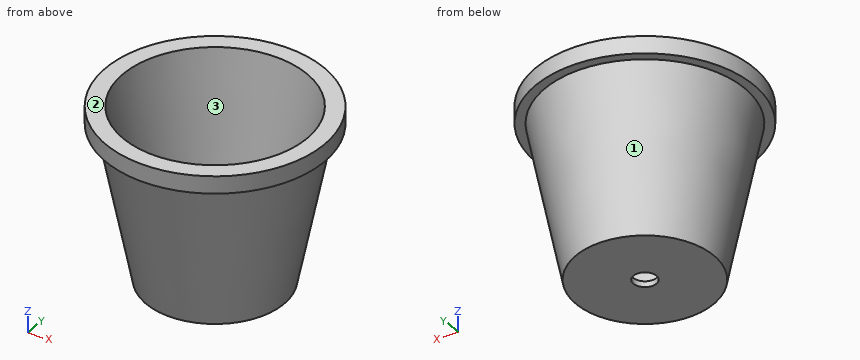
```python
from build123d import *

# Parameters (mm, degrees)
SKETCH_R      = 10
POCKET_DEPTH  = 5
SKETCH001_R   = 95
SKETCH001_R_2 = 82.96172
PAD_DEPTH     = 15


with BuildPart() as kegel001:
    # Cone001 → Cone001 (revolve)
    with BuildSketch(Plane(origin=(0, 0, 5), x_dir=(1, 0, 0), z_dir=(0, -1, 0))):
        Polygon((0, 0), (50, 0), (80, 145), (0, 145), align=None)
    revolve(axis=Axis((0, 0, 5), (0, 0, 1)))


with BuildPart() as pocket:
    # Cone → Cone (revolve)
    with BuildSketch(Plane.XZ):
        Polygon((0, 0), (60, 0), (90, 150), (0, 150), align=None)
    revolve(axis=Axis((0, 0, 0), (0, 0, 1)))

    # Cut: cut Kegel001
    add(kegel001.part, mode=Mode.SUBTRACT)

    # Sketch → Pocket (cut)
    with BuildSketch(Plane(origin=(0, 0, 0), x_dir=(1, 0, 0), z_dir=(0, 0, -1))):
        Circle(SKETCH_R)
    extrude(amount=-POCKET_DEPTH, mode=Mode.SUBTRACT)


with BuildPart() as obj1:
    # Sketch001 → Pad (new body)
    with BuildSketch(Plane.XY.offset(150)):
        Circle(SKETCH001_R)
        Circle(SKETCH001_R_2, mode=Mode.SUBTRACT)
    extrude(amount=-PAD_DEPTH)

    # Fusion: union Pocket
    add(pocket.part)


solid = obj1.part
```
Geometry check sheet. Reference: the model listing, model coordinates, mm. Face numbers are marked on the shaded views. Coordinates: 2 decimals unless noted, no trailing zeros. Order: outer loops, then holes, each group sorted by start corner. A loop starts at its lowest first (then second) coordinate and runs counter-clockwise, first axis right, second up.
Item 1: Section check A-A (y = 0). Enter the section's corners in (x, z).
Item 2: Mould release check, pull along Y, two halves, no side actions. Record for the marked faces 1, 2 and 3: released by +Y, released by -Y, zero draft, split by the parting line, or undercut.
Item 3: Scan lines: line 1 along Z through (x, y) = (28.5, -10); line 2 along Y through (x, z) = (0, 3); line 3 along Y through (x, z) = (0, 4.05). Record each from-to range of solid material in increasing order.
Item 4: Section check C-C (z = 61). Enter the section's corners in (x, y), plus the area to 3 significant figures.
Item 5: Depth check by flat-ended pin: pin 1 (6 mm diameter, centred on y = 16.5, z = 19, fed in from +X); pin 2 (1 mm diameter, centred on x = -31, y = -11, fed in from +Z); pin 3 (18 mm diameter, centred on x = 0, y = 0, fed in from +Z); pin 4 (1.5 mm diameter, centred on y = -2, z = 126, fed in from +X). Enter the tip coordinate at first touch or a pass-through.
Check sheet entries:
1. outline: (-95, 135) - (-87, 135) - (-60, 0) - (-10, 0) - (-10, 5) - (-50, 5) - (-80, 150) - (-95, 150) - close; (10, 0) - (60, 0) - (87, 135) - (95, 135) - (95, 150) - (80, 150) - (50, 5) - (10, 5) - close
2. face 1: split by the parting line
2. face 2: zero draft
2. face 3: undercut
3. line 1: z = 0 to 5
3. line 2: y = -60.6 to -10, 10 to 60.6
3. line 3: y = -60.81 to -10, 10 to 60.81
4. outline: circle Ø144.4 at (0, 0); hole circle Ø123.17 at (0, 0)
4. area: 4,460 mm2
5. pin 1: stops at x = 62.6
5. pin 2: stops at z = 5
5. pin 3: passes through
5. pin 4: stops at x = 85.33
